```python
from build123d import *

# Parameters (mm, degrees)
F0_W        = 21
F0_H        = 12
F0_R        = 1.75
F1_DEPTH    = 3
F2_W        = 2.9
F2_H        = 12
F3_DEPTH    = 10
F4_R        = 2
F5_DEPTH    = 21.001
F6_T1_DEPTH = 43
F7_SIZE     = 1
F8_R        = 4
F9_R        = 0.5
F10_R       = 3.5
F11_DEPTH   = 0.8
F13_DEPTH   = 1.2


# Not quite as in the source:
# - a fillet or chamfer that OpenCascade refuses, or shapes differently, is made with other operations: its cross-section is extruded or revolved along the edge and cut away or added


with BuildPart() as f1:
    # F0 (on Top) → F1 (new body)
    with BuildSketch(Plane.XY):
        with Locations((10.5, 6)):
            Rectangle(F0_W, F0_H)
        with Locations((6, 6)):
            Circle(F0_R, mode=Mode.SUBTRACT)
        with Locations((15, 6)):
            Circle(F0_R, mode=Mode.SUBTRACT)
    extrude(amount=F1_DEPTH)

    # F2 (on face) → F3 (join)
    with BuildSketch(Plane.XY.offset(3)):
        with Locations((1.45, 6)):
            Rectangle(F2_W, F2_H)
        with Locations((19.55, 6)):
            Rectangle(F2_W, F2_H)
    extrude(amount=F3_DEPTH)

    # F4 (on face) → F5 (cut, through all)
    with BuildSketch(Plane(origin=(0, 0, 0), x_dir=(0, -1, 0), z_dir=(-1, 0, 0))):
        with Locations((-6, 9)):
            Circle(F4_R)
    extrude(amount=-F5_DEPTH, mode=Mode.SUBTRACT)

    # F6: fillet of radius 6 on 1 edges, made by hand

    # F6_s2 → F6_t1 (cut)
    with BuildSketch(Plane.XY.offset(-15)):
        with BuildLine():
            ThreePointArc((15, 0), (19.2426406871, 1.7573593129), (21, 6))
            Line((21, 6), (21, 0))
            Line((21, 0), (15, 0))
        make_face()
    extrude(amount=F6_T1_DEPTH, mode=Mode.SUBTRACT)

    # F7
    f7_edges = [f1.edges().sort_by_distance(p)[0] for p in [
        (8.95, 0, 3),
        (10.5, 12, 3),
    ]]
    chamfer(f7_edges, length=F7_SIZE)

    # F8
    f8_edges = [f1.edges().sort_by_distance(p)[0] for p in [
        (19.55, 12, 13),
        (1.45, 0, 13),
        (1.45, 12, 13),
    ]]
    fillet(f8_edges, radius=F8_R)

    # F9
    f9_edges = [f1.edges().sort_by_distance(p)[0] for p in [
        (18.1, 0.86288, 8),
    ]]
    fillet(f9_edges, radius=F9_R)

    # F10 (on face) → F11 (cut)
    with BuildSketch(Plane.YZ.offset(21)):
        with Locations((6, 9)):
            Circle(F10_R)
    extrude(amount=-F11_DEPTH, mode=Mode.SUBTRACT)

    # F12 (on face) → F13 (cut)
    with BuildSketch(Plane(origin=(0, 0, 0), x_dir=(0, -1, 0), z_dir=(-1, 0, 0))):
        Polygon((-3.15, 7.3545517328), (-3.15, 10.6454482672), (-6, 12.2908965344), (-8.85, 10.6454482672), (-8.85, 7.3545517328), (-6, 5.7091034656), align=None)
    extrude(amount=-F13_DEPTH, mode=Mode.SUBTRACT)


solid = f1.part
```
Input: part model. Units: mm. Frame: model coordinates. A direction names the side the tool comes from. Coordinates: 2 decimals unless noted, no trailing zeros. Write each loop counter-clockwise with the first axis right and the second up, starting at its lowest first coordinate (ties: lowest second). Pieces come first, ordered by that corner, then holes. Notation, with made-up numbers: (-32.5, 20) -> (7.5, 20) arc R13 cw to (7.5, 41) -> close; hole circle Ø5 at (68, 40). An arc over 180 degrees is marked (long way). Answer as a JSON object with one key per item and string values.
1. Section B-B on y = 5.5. Count the separate pieces of the cut face and the enclosed holes in it, then the cut area to 3 significant figures.
Result set:
{"separate pieces": "5", "enclosed holes": "0", "area": "73.3 mm2"}
2. Mould query, pull axis X, two halves, no side actions, for faces 1 (the face through (19.57, 10.859, 11.797)), 2 (the face through (10, 6, 3)), 3 (the face through (0, 6, 5)), 4 (the face through (20.2, 8, 7)). Classes: released by +X, released by -X, zero draft, split by the parting line, or undercut.
Result set:
{"face 1": "zero draft", "face 2": "undercut", "face 3": "released by -X", "face 4": "released by +X"}
3. Section A-A on x = 6. Return the cut outline in (y, z), then the cut area to 3 significant figures.
Result set:
{"outline": "(0, 0) -> (4.25, 0) -> (4.25, 3) -> (1, 3) -> (0, 2) -> close; (7.75, 0) -> (12, 0) -> (12, 2) -> (11, 3) -> (7.75, 3) -> close", "area": "24.5 mm2"}
4. First-contact query: P1, Ø2, axis at x = 13.5, y = 10.5, coming from the +Z side; P2, Ø4.5, axis at y = 6, z = 9, coming from the -X side; P3, Ø5.5, axis at y = 8, z = 7.5, coming from the +X side; P4, Ø3, axis at x = 6, y = 6, coming from the +Z side. Flat tips, straight axial feed; report the tip coordinate or a pass-through.
Result set:
{"P1": "stops at z = 3", "P2": "stops at x = 1.2", "P3": "stops at x = 21", "P4": "passes through"}
5. Section C-C on z = 4. Return the cut outline in (x, y).
Result set:
{"outline": "(0, 0) -> (2.9, 0) -> (2.9, 12) -> (0, 12) -> close; (18.1, 1.84) arc R0.5 ccw to (18.93, 1.46) arc R6 ccw to (21, 6) -> (21, 12) -> (18.1, 12) -> close"}
6. Access query for faces 5 (the face through (1.2, 8, 8)), 6 (the face through (10.4, 11.5, 2.5)), 7 (the face through (18.399, 1.384, 7.423)), 8 (the face through (20.6, 9.5, 8.9)). Directions: +Z, -Z, +X, -X, +Y, -Y. A direction counts if a zero-diameter tool reaches every point of the face in a straight line with its end or side. Return the directions, or none.
Result set:
{"face 5": "-X", "face 6": "+Z, +Y", "face 7": "+Z, -Y", "face 8": "+X"}
7. Section D-D on x = 11.5. Return the cut outline in (y, z).
Result set:
{"outline": "(0, 0) -> (12, 0) -> (12, 2) -> (11, 3) -> (1, 3) -> (0, 2) -> close"}
8. Material intervals for line 1 (X direction, y = 8.5, z = 6.5); line 2 (Y direction, x = 15, z = 1.65); line 3 (X direction, y = 3, z = 11.5), sorted ascending. Write a range as from..to.
Result set:
{"line 1": "x = 0..2.9, 18.1..21", "line 2": "y = 0..4.25, 7.75..12", "line 3": "x = 0..2.9, 18.1..20.2"}
